Geometry check sheet. Reference: the model listing, model coordinates, mm. Round coordinates to 2 decimals unless told otherwise and drop trailing zeros. Write each loop counter-clockwise with the first axis right and the second up, starting at its lowest first coordinate (ties: lowest second). Pieces come first, ordered by that corner, then holes.
Item 1: Cross-section at A-A (x = -1.5). Enter the section's corners in (y, z).
Item 2: Cross-section at B-B (z = 0.55). Enter the section's corners in (x, y), then the cut area to 3 significant figures.
Item 3: Cross-section at D-D (x = -7.25). Enter the section's corners in (y, z), then the cut area to 3 significant figures.
Item 4: Scan lines: probe 1 along X at (y, z) = (-16.25, 0.4); probe 2 along Y at (x, z) = (-4.5, 0.6); probe 3 along X at (y, z) = (-14.5, 0.75). Record each from-to range of solid material in increasing order.
Item 5: Cross-section at C-C (y = -24.25). Enter the section's corners in (x, z).
Item 6: Draft check along X on faces 1 (the face through (-1.475, -19.547, 0.493)), 2 (the face through (-7.855, -11.648, 0.493)), 3 (the face through (-2.5, -27.6, 0.5)). Enter one of: pulls with the +X half, pulls with the -X half, needs draft (parallel to the pull), parting line crosses it, or undercut.
Autodesk Inventor part; units mm, degrees
ref_plane "YZ Plane" through (0, 0, 0) normal (1, 0, 0) x (0, 1, 0)
ref_plane "XZ Plane" through (0, 0, 0) normal (0, 1, 0) x (-1, 0, 0)
ref_plane "XY Plane" through (0, 0, 0) normal (0, 0, 1) x (1, 0, 0)
sketch "Sketch1" plane through (0, 0, 0) normal (0, 0, 1) x (1, 0, 0)
  line L0 (-1.9526, -19.2383) -> (-0.4726, -26.9699)
  line L1 (-1.0107, -19.8473) -> (-1.9526, -19.2383)
  arc A0 (0.7413, -3.1056) -> (-1.0107, -19.8473) centre (49.2329, -16.6427) ccw
  line L2 (-3.5931, -0.3031) -> (0.7413, -3.1056)
  arc A1 (-3.5931, -0.3031) -> (-7.7014, -23.436) centre (23.9637, -17.1282) ccw
  arc A2 (-4.6851, -27.4777) -> (-7.7014, -23.436) centre (-10.5765, -28.728) ccw
  arc A3 (-4.6851, -27.4777) -> (-0.4726, -26.9699) centre (-3.2557, -21.6091) ccw
extrude "Extrusion1" add sketch "Sketch1" along normal blind 1
properties part number "cueromango"
Resolved:
1. outline: (-27.39, 0) - (-21.6, 0) - (-21.6, 1) - (-27.39, 1) - close; (-19.53, 0) - (-1.66, 0) - (-1.66, 1) - (-19.53, 1) - close
2. outline: (-7.7, -23.44) arc R6.02 cw to (-4.69, -27.48) arc R6.04 ccw to (-0.47, -26.97) - (-1.95, -19.24) - (-1.01, -19.85) arc R50.35 cw to (0.74, -3.11) - (-3.59, -0.3) arc R32.29 ccw to start
2. area: 166 mm2
3. outline: (-23.71, 0) - (-8.87, 0) - (-8.87, 1) - (-23.71, 1) - close
3. area: 14.8 mm2
4. probe 1: x = -8.31 to -1.11
4. probe 2: y = -27.52 to -1.89
4. probe 3: x = -8.22 to -1.07
5. outline: (-6.55, 0) - (-0.99, 0) - (-0.99, 1) - (-6.55, 1) - close
6. face 1: undercut
6. face 2: pulls with the -X half
6. face 3: parting line crosses it
